Verification items for this drawing (mm, ordinates from the low corner). A direction names the side the tool comes from. Round coordinates to 2 decimals unless told otherwise and drop trailing zeros. Order: outer loops, then holes, each group sorted by start corner. A loop starts at its lowest first (then second) coordinate and runs counter-clockwise, first axis right, second up. Notation, with made-up numbers: M 75.25,13.5 L 80.25,13.5 A9 cw 80.25,28.5 Z; hole C 86.25,53.25 d1. An arc over 180 degrees is marked long. One line per item, written item: value. Start each with the question number.
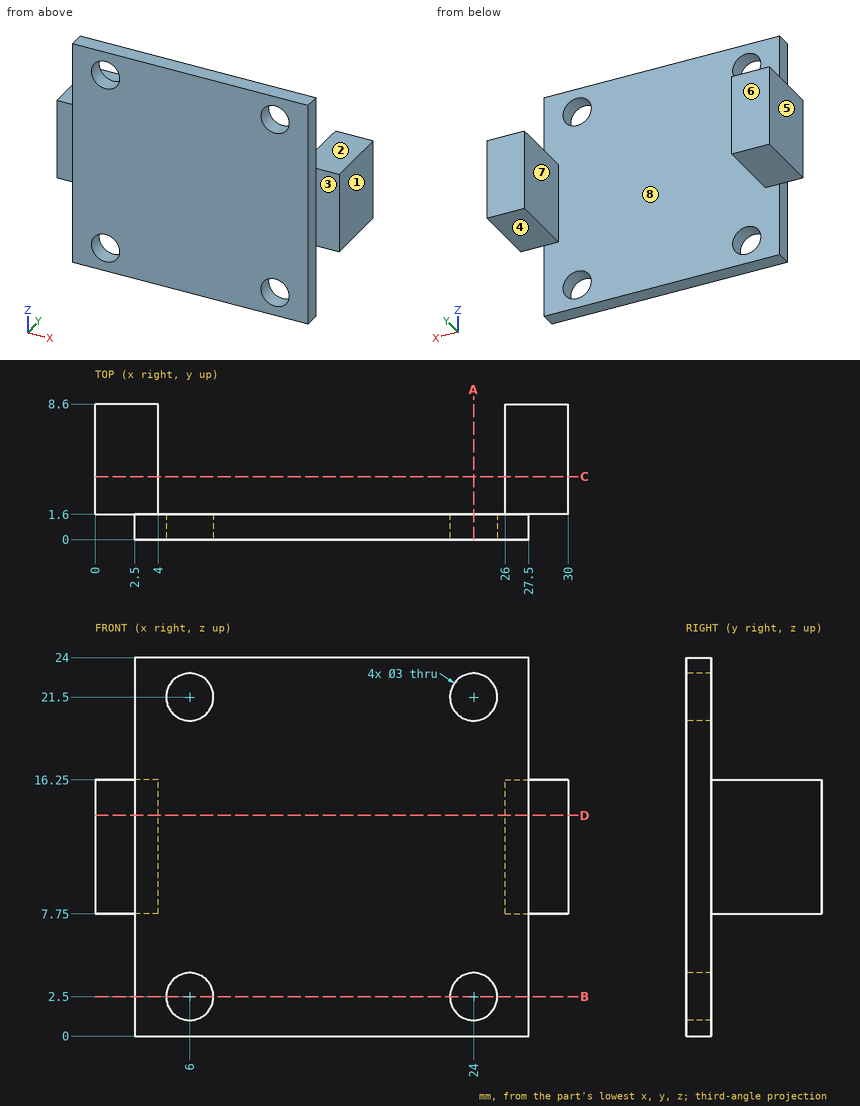
1. Tool access check on the marked faces 1, 2, 3 and 4. Record the directions out of +Z, -Z, +X, -X, +Y, -Y that give a thin tool (end or side, any length) a straight path to the whole face; none if there is none.
2. Section check C-C (y = 4). Record the cut outline in (x, z).
3. Section check A-A (x = 24). Record the cut outline in (y, z).
4. Scan lines: line 1 along Z through (x, y) = (24, 1.05); line 2 along X through (y, z) = (0.8, 2.5); line 3 along X through (y, z) = (2.5, 14.75). Record each from-to range of solid material in increasing order.
5. Section check B-B (z = 2.5). Record the cut outline in (x, y).
6. Section check D-D (z = 14). Record the cut outline in (x, y).
7. Draft check along X on the marked faces 5, 6, 7 and 8. Enter one of: released by +X, released by -X, zero draft, split by the parting line, or undercut.
8. Depth check by flat-ended pin: pin 1 (4 mm diameter, centred on x = 6, z = 2.5, fed in from +Y); pin 2 (2.5 mm diameter, centred on x = 24, z = 21.5, fed in from +Y); pin 3 (4.5 mm diameter, centred on x = 28.5, y = 4, fed in from -Z); pin 4 (3 mm diameter, centred on x = 2, y = 6.5, fed in from +Z). Enter the tip coordinate at first touch or a pass-through.
Geometry check:
1. face 1: +Z, -Z, +X, +Y, -Y
1. face 2: +Z, +X, -X, +Y
1. face 3: +Z, -Z, +X, -Y
1. face 4: -Z, +X, -X, +Y
2. outline: M 0,7.75 L 4,7.75 L 4,16.25 L 0,16.25 Z; M 26,7.75 L 30,7.75 L 30,16.25 L 26,16.25 Z
3. outline: M 0,0 L 1.6,0 L 1.6,1 L 0,1 Z; M 0,4 L 1.6,4 L 1.6,20 L 0,20 Z; M 0,23 L 1.6,23 L 1.6,24 L 0,24 Z
4. line 1: z = 0 to 1, 4 to 20, 23 to 24
4. line 2: x = 2.5 to 4.5, 7.5 to 22.5, 25.5 to 27.5
4. line 3: x = 0 to 4, 26 to 30
5. outline: M 2.5,0 L 4.5,0 L 4.5,1.6 L 2.5,1.6 Z; M 7.5,0 L 22.5,0 L 22.5,1.6 L 7.5,1.6 Z; M 25.5,0 L 27.5,0 L 27.5,1.6 L 25.5,1.6 Z
6. outline: M 0,1.6 L 2.5,1.6 L 2.5,0 L 27.5,0 L 27.5,1.6 L 30,1.6 L 30,8.6 L 26,8.6 L 26,1.6 L 4,1.6 L 4,8.6 L 0,8.6 Z
7. face 5: released by -X
7. face 6: zero draft
7. face 7: undercut
7. face 8: undercut
8. pin 1: stops at y = 1.6
8. pin 2: passes through
8. pin 3: stops at z = 7.75
8. pin 4: stops at z = 16.25
